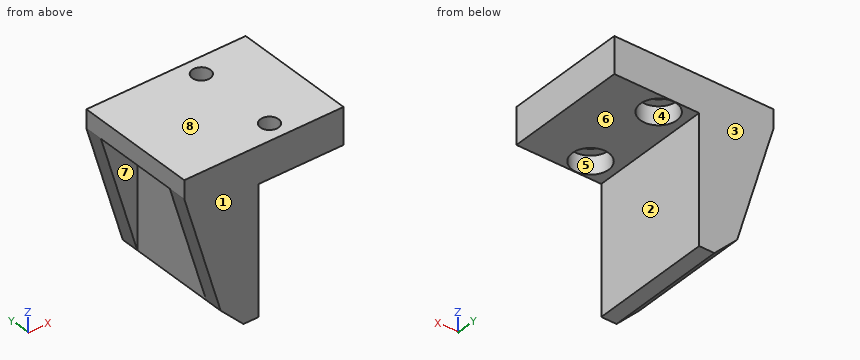
```python
from build123d import *

# Parameters (mm, degrees)
SKETCH1_W           = 17.145
SKETCH1_H           = 17.145
BOSS_EXTRUDE1_DEPTH = 5.08
SKETCH2_R           = 1.27
CUT_EXTRUDE1_DEPTH  = 6.08
SKETCH3_R           = 2.54
CUT_EXTRUDE4_DEPTH  = 2.54
SKETCH4_W           = 6.307704678
SKETCH4_H           = 17.145
BOSS_EXTRUDE2_DEPTH = 17.78
SKETCH5_W           = 2.54
SKETCH5_H           = 17.145
BOSS_EXTRUDE3_DEPTH = 5.08
CHAMFER1_SIZE       = 3.175
BOSS_EXTRUDE4_DEPTH = 2.54
BOSS_EXTRUDE5_DEPTH = 2.54
SKETCH9_W           = 1
SKETCH9_H           = 17.145
CUT_EXTRUDE5_DEPTH  = 17.78


with BuildPart() as part:
    # Sketch1 → Boss-Extrude1 (new body)
    with BuildSketch(Plane.XY):
        with Locations((8.5725, -8.5725)):
            Rectangle(SKETCH1_W, SKETCH1_H)
    extrude(amount=BOSS_EXTRUDE1_DEPTH)

    # Sketch2 → Cut-Extrude1 (cut, through all)
    with BuildSketch(Plane(origin=(0, 0, 0), x_dir=(-1, 0, 0), z_dir=(0, 0, -1))):
        with Locations((-8.89, -2.5908)):
            Circle(SKETCH2_R)
        with Locations((-8.89, -14.5288)):
            Circle(SKETCH2_R)
    extrude(amount=-CUT_EXTRUDE1_DEPTH, mode=Mode.SUBTRACT)

    # Sketch3 → Cut-Extrude4 (cut)
    with BuildSketch(Plane(origin=(0, 0, 0), x_dir=(-1, 0, 0), z_dir=(0, 0, -1))):
        with Locations((-8.89, -2.5908)):
            Circle(SKETCH3_R)
        with Locations((-8.89, -14.5288)):
            Circle(SKETCH3_R)
    extrude(amount=-CUT_EXTRUDE4_DEPTH, mode=Mode.SUBTRACT)

    # Sketch4 → Boss-Extrude2 (add)
    with BuildSketch(Plane(origin=(0, 0, 0), x_dir=(-1, 0, 0), z_dir=(0, 0, -1))):
        with Locations((-3.153852339, -8.5725)):
            Rectangle(SKETCH4_W, SKETCH4_H)
    extrude(amount=BOSS_EXTRUDE2_DEPTH)

    # Sketch5 → Boss-Extrude3 (add)
    with BuildSketch(Plane.ZY):
        with Locations((3.81, -8.5725)):
            Rectangle(SKETCH5_W, SKETCH5_H)
    extrude(amount=BOSS_EXTRUDE3_DEPTH)

    # Chamfer1
    chamfer1_edges = [part.edges().sort_by_distance(p)[0] for p in [
        (0, -8.5725, -17.78),
    ]]
    chamfer(chamfer1_edges, length=CHAMFER1_SIZE)

    # Sketch7 → Boss-Extrude4 (add)
    with BuildSketch(Plane(origin=(0, 0, 0), x_dir=(1, 0, 0), z_dir=(0, 1, 0))):
        Polygon((-5.08, -2.54), (0, 14.605), (0, -2.54), align=None)
    extrude(amount=-BOSS_EXTRUDE4_DEPTH)

    # Sketch8 → Boss-Extrude5 (add)
    with BuildSketch(Plane.XZ.offset(17.145)):
        Polygon((0, 2.54), (-5.08, 2.54), (0, -14.605), align=None)
    extrude(amount=-BOSS_EXTRUDE5_DEPTH)

    # Sketch9 → Cut-Extrude5 (cut)
    with BuildSketch(Plane(origin=(0, 0, -17.78), x_dir=(-1, 0, 0), z_dir=(0, 0, -1))):
        with Locations((-5.807704678, -8.5725)):
            Rectangle(SKETCH9_W, SKETCH9_H)
    extrude(amount=-CUT_EXTRUDE5_DEPTH, mode=Mode.SUBTRACT)


solid = part.part
```
Source: CAD feature listing. Evaluate the final solid. Frame: model axes, mm. Face numbers are marked on the shaded views. A direction names the side the tool comes from. Coordinates: 2 decimals unless noted, no trailing zeros. Write each loop counter-clockwise with the first axis right and the second up, starting at its lowest first coordinate (ties: lowest second). Pieces come first, ordered by that corner, then holes. Notation, with made-up numbers: M 33,89 L 85,89 A12 cw 85,100 Z; hole C 46.25,53 d6. An arc over 180 degrees is marked long. Answer as a JSON object with one key per item and string values.
1. Ray query, L1, parallel to Y at x = 8.89, z = 3.1 (3 decimals); L2, parallel to Z at x = 12, y = -10.75; L3, parallel to Z at x = -1, y = -3. Return the intervals inside material, ascending.
Evaluation:
{"L1": "-17.145 to -15.799, -13.259 to -3.861, -1.321 to 0", "L2": "0 to 5.08", "L3": "2.54 to 5.08"}
2. Cut plane B-B on z = -11.5. Output: boundary loops of the cut face in (x, y) (3 decimals).
Evaluation:
{"outline": "M -0.92,-17.145 L 5.308,-17.145 L 5.308,0 L -0.92,0 L -0.92,-2.54 L 0,-2.54 L 0,-14.605 L -0.92,-14.605 Z"}
3. Cut plane C-C on y = -10.75. Output: boundary loops of the cut face in (x, z) (3 decimals), plus the area to 3 significant figures.
Evaluation:
{"outline": "M -5.08,2.54 L 0,2.54 L 0,-14.605 L 3.175,-17.78 L 5.308,-17.78 L 5.308,0 L 17.145,0 L 17.145,5.08 L -5.08,5.08 Z", "area": "189 mm^2"}
4. Contact query for flat-ended pins moving along their axis: P1, Ø1.5, axis at y = -4, z = -15.5, coming from the -X side (3 decimals); P2, Ø6, axis at x = 12.5, y = -10.5, coming from the -Z side; P3, Ø10, axis at y = -11.5, z = -8.5, coming from the +X side; P4, Ø2.5, axis at x = -3.5, z = -8.5, coming from the -Y side. Output: stop coordinate, or through.
Evaluation:
{"P1": "x = 0.145", "P2": "z = 0", "P3": "x = 5.31", "P4": "through"}
5. Draft query along Y for the marked faces 1, 2, 3 and 4. Return one class per face: released by +Y, released by -Y, zero draft, split by the parting line, or undercut.
Evaluation:
{"face 1": "released by -Y", "face 2": "zero draft", "face 3": "released by +Y", "face 4": "undercut"}
6. Cut plane A-A on x = 8.89. Output: boundary loops of the cut face in (y, z) (3 decimals).
Evaluation:
{"outline": "M -17.145,0 L -17.069,0 L -17.069,2.54 L -15.799,2.54 L -15.799,5.08 L -17.145,5.08 Z; M -13.259,2.54 L -11.989,2.54 L -11.989,0 L -5.131,0 L -5.131,2.54 L -3.861,2.54 L -3.861,5.08 L -13.259,5.08 Z; M -1.321,2.54 L -0.051,2.54 L -0.051,0 L 0,0 L 0,5.08 L -1.321,5.08 Z"}
7. Cut plane D-D on x = 13. Output: boundary loops of the cut face in (y, z) (3 decimals), plus the area to 3 significant figures.
Evaluation:
{"outline": "M -17.145,0 L 0,0 L 0,5.08 L -17.145,5.08 Z", "area": "87.1 mm^2"}
8. Access query for the marked faces 5, 6, 7 and 8. Directions: +Z, -Z, +X, -X, +Y, -Y. A direction counts if a zero-diameter tool reaches every point of the face in a straight line with its end or side. Return the directions, or none.
Evaluation:
{"face 5": "-Z", "face 6": "-Z, +X, +Y, -Y", "face 7": "-Z, -X", "face 8": "+Z, +X, -X, +Y, -Y"}
